```python
from build123d import *

# Parameters (mm, degrees)
SKETCH1_W            = 63.5
SKETCH1_H            = 20
SKETCH1_R            = 1.4
BASE_DEPTH           = 5
F_1MM_EDGE_FILLETS_R = 1


with BuildPart() as part:
    # Sketch1 → Base (new body)
    with BuildSketch(Plane(origin=(0, 0, 0), x_dir=(1, 0, 0), z_dir=(0, 1, 0))):
        Rectangle(SKETCH1_W, SKETCH1_H)
        with Locations(Location((-25.25, 0, 0), (0, 0, 270))):
            Circle(SKETCH1_R, mode=Mode.SUBTRACT)
        with Locations(Location((25.25, 0, 0), (0, 0, 90))):
            Circle(SKETCH1_R, mode=Mode.SUBTRACT)
    extrude(amount=BASE_DEPTH)

    # 1mm Edge Fillets
    f_1mm_edge_fillets_edges = [part.edges().sort_by_distance(p)[0] for p in [
        (31.75, 5, 0),
        (0, 5, -10),
        (-31.75, 5, 0),
        (-31.75, 2.5, -10),
        (31.75, 2.5, -10),
        (31.75, 2.5, 10),
        (-31.75, 2.5, 10),
        (0, 5, 10),
    ]]
    fillet(f_1mm_edge_fillets_edges, radius=F_1MM_EDGE_FILLETS_R)


solid = part.part
```
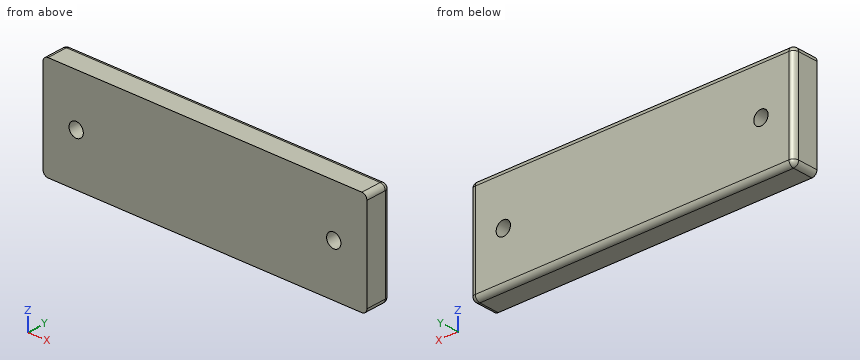
Model file for the job. Use its own axes, mm. Round coordinates to 2 decimals unless told otherwise and drop trailing zeros. Loops run counter-clockwise (first coordinate to the right, second up) from the corner with the lowest first, then second, coordinate; pieces in that order, holes last. Notation, with made-up numbers: M 43,14.5 L 93,14.5 A23 cw 93,39.5 Z; hole C 89.5,56 d6. An arc over 180 degrees is marked long. Put each result on its own line as item: value. Start each with the question number.
Item 1: Drill centre lines: line 1 along X through (y, z) = (2.2, 0); line 2 along Z through (x, y) = (25.25, 3.5); line 3 along Y through (x, z) = (2.5, 9.25). Where is each one in solid material? Low to high.
Item 2: Cut at C-C (x = 26). List the corners of the cut face in (y, z), then the cut area to 3 significant figures.
Item 3: Cut at A-A (x = -25.25). List the corners of the cut face in (y, z).
Item 4: Cut at B-B (z = 0). List the corners of the cut face in (x, y), then the cut area to 3 significant figures.
Answer block:
1. line 1: -31.75 to -26.65, -23.85 to 23.85, 26.65 to 31.75
1. line 2: -10 to -1.4, 1.4 to 10
1. line 3: 0 to 4.97
2. outline: M 0,-10 L 4,-10 A1 ccw 5,-9 L 5,-1.18 L 0,-1.18 Z; M 0,1.18 L 5,1.18 L 5,9 A1 ccw 4,10 L 0,10 Z
2. area: 87.7 mm2
3. outline: M 0,-10 L 4,-10 A1 ccw 5,-9 L 5,-1.4 L 0,-1.4 Z; M 0,1.4 L 5,1.4 L 5,9 A1 ccw 4,10 L 0,10 Z
4. outline: M -31.75,0 L -26.65,0 L -26.65,5 L -30.75,5 A1 ccw -31.75,4 Z; M -23.85,0 L 23.85,0 L 23.85,5 L -23.85,5 Z; M 26.65,0 L 31.75,0 L 31.75,4 A1 ccw 30.75,5 L 26.65,5 Z
4. area: 289 mm2
